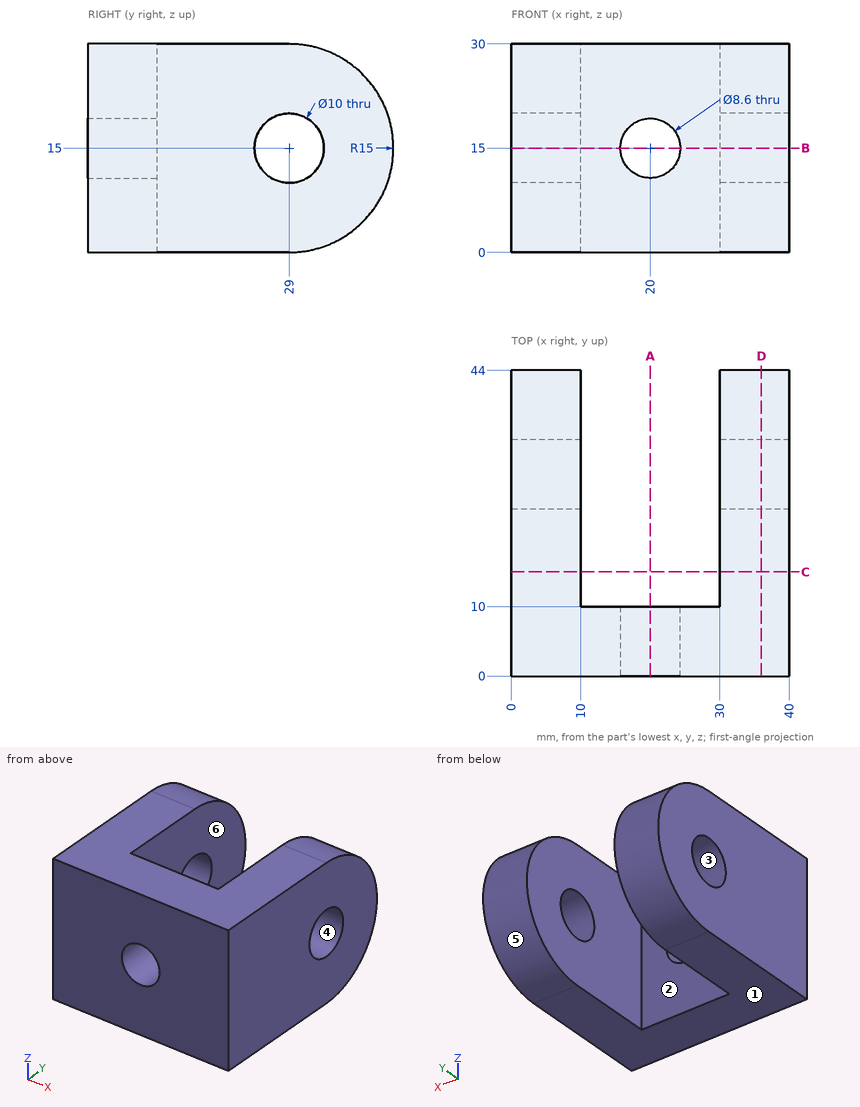
Geometry: see drawing. Coordinates: mm, zero at the bounding-box minimum. A direction names the side the tool comes from. Give positions to 0.01 mm unless a question says otherwise; leave off trailing zeros. Order: outer loops, then holes, each group sorted by start corner. A loop starts at its lowest first (then second) coordinate and runs counter-clockwise, first axis right, second up. Notation, with made-up numbers: (1.5, 50) -> (21.5, 50) arc R14 cw to (21.5, 71) -> close; hole circle Ø7 at (77, 81.5). An arc over 180 degrees is marked (long way). Write each question's results on one line, items separated by ' | '.
1) First-contact query: pin 1 Ø6 at (x, z) = (6.5, 11.5) entering from +Y; pin 2 Ø6 at (y, z) = (29, 15) entering from -X; pin 3 Ø3 at (x, z) = (34.5, 10) entering from +Y. Flat tips, straight axial feed; report the tip coordinate or a pass-through.
Geometry says:
pin 1: stops at y = 43.99 | pin 2: passes through | pin 3: stops at y = 43.59
2) Cut plane C-C (y = 15). Output: boundary loops of the cut face in (x, z), and give its area (3 significant figures).
Geometry says:
outline: (0, 0) -> (10, 0) -> (10, 30) -> (0, 30) -> close; (30, 0) -> (40, 0) -> (40, 30) -> (30, 30) -> close | area: 600 mm²
3) Line query: line 1 along X through (y, z) = (23.5, 19); line 2 along Y through (x, z) = (37.5, 15); line 3 along Z through (x, y) = (20, 5). Output: solid intervals per line, ascending.
Geometry says:
line 1: x = 0 to 10, 30 to 40 | line 2: y = 0 to 24, 34 to 44 | line 3: z = 0 to 10.7, 19.3 to 30
4) Draft query along Z for the marked faces 1, 2, 3 and 4. Return one class per face: released by +Z, released by -Z, zero draft, split by the parting line, or undercut.
Geometry says:
face 1: released by -Z | face 2: zero draft | face 3: undercut | face 4: undercut
5) Cut plane D-D (x = 36). Output: boundary loops of the cut face in (y, z).
Geometry says:
outline: (0, 0) -> (29, 0) arc R15 ccw to (29, 30) -> (0, 30) -> close; hole circle Ø10 at (29, 15)
6) Cut plane A-A (x = 20). Output: boundary loops of the cut face in (y, z), and give its area (3 significant figures).
Geometry says:
outline: (0, 0) -> (10, 0) -> (10, 10.7) -> (0, 10.7) -> close; (0, 19.3) -> (10, 19.3) -> (10, 30) -> (0, 30) -> close | area: 214 mm²
7) Cut plane B-B (z = 15). Output: boundary loops of the cut face in (x, y), and give its area (3 significant figures).
Geometry says:
outline: (0, 0) -> (15.7, 0) -> (15.7, 10) -> (10, 10) -> (10, 24) -> (0, 24) -> close; (0, 34) -> (10, 34) -> (10, 44) -> (0, 44) -> close; (24.3, 0) -> (40, 0) -> (40, 24) -> (30, 24) -> (30, 10) -> (24.3, 10) -> close; (30, 34) -> (40, 34) -> (40, 44) -> (30, 44) -> close | area: 794 mm²
8) Set-up query: the marked faces 5 and 6. Return all of +Z, -Z, +X, -X, +Y, -Y with unobstructed straight access to the full face (end or side cutting, diameter ignored); none if empty.
Geometry says:
face 5: +X, -X, +Y | face 6: +Z, -Z, +Y
